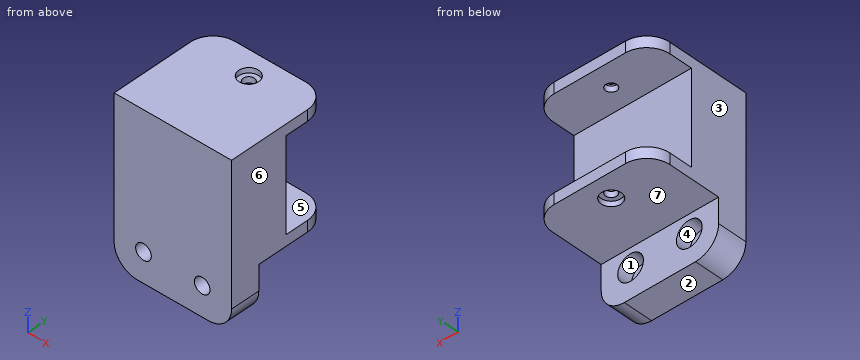
```python
from build123d import *

# Parameters (mm, degrees)
SKETCH1_W                                        = 50.8
SKETCH1_H                                        = 25.4
BOSS_EXTRUDE1_DEPTH                              = 25.4
CBORE_FOR_1_4_SOCKET_HEAD_CAP_SCREW1_D           = 6.7564
CBORE_FOR_1_4_SOCKET_HEAD_CAP_SCREW1_CBORE_D     = 11.1125
CBORE_FOR_1_4_SOCKET_HEAD_CAP_SCREW1_CBORE_DEPTH = 19.05
SKETCH6_W                                        = 50.8
SKETCH6_H                                        = 4.7
BOSS_EXTRUDE2_DEPTH                              = 20
CBORE_FOR_M4_SBHCS1_D                            = 4.8
CBORE_FOR_M4_SBHCS1_CBORE_D                      = 8.6
CBORE_FOR_M4_SBHCS1_CBORE_DEPTH                  = 2.2
FILLET1_R                                        = 10
SKETCH15_W                                       = 50.8
SKETCH15_H                                       = 25.4
BOSS_EXTRUDE3_DEPTH                              = 20
SKETCH16_W                                       = 51.113320751
SKETCH16_H                                       = 27.993322013
CUT_EXTRUDE2_DEPTH                               = 12.7
SKETCH17_W                                       = 50.8
SKETCH17_H                                       = 12.7
CUT_EXTRUDE3_DEPTH                               = 20.7


with BuildPart() as part:
    # Sketch1 → Boss-Extrude1 (new body)
    with BuildSketch(Plane(origin=(0, 0, 0), x_dir=(1, 0, 0), z_dir=(0, 1, 0))):
        with Locations((2.315568022, 7.890743338)):
            Rectangle(SKETCH1_W, SKETCH1_H)
    extrude(amount=BOSS_EXTRUDE1_DEPTH)

    # CBORE for 1/4 Socket Head Cap Screw1 (through all)
    with Locations(Plane(origin=(0, 25.4, 0), x_dir=(1, 0, 0), z_dir=(0, 1, 0))):
        with Locations((-10.384431978, 7.890743338), (15.015568022, 7.890743338)):
            CounterBoreHole(CBORE_FOR_1_4_SOCKET_HEAD_CAP_SCREW1_D / 2, CBORE_FOR_1_4_SOCKET_HEAD_CAP_SCREW1_CBORE_D / 2, CBORE_FOR_1_4_SOCKET_HEAD_CAP_SCREW1_CBORE_DEPTH)

    # Sketch6 → Boss-Extrude2 (add)
    with BuildSketch(Plane(origin=(0, 25.4, 0), x_dir=(1, 0, 0), z_dir=(0, 1, 0))):
        with Locations((2.315568022, 18.240743338)):
            Rectangle(SKETCH6_W, SKETCH6_H)
    extrude(amount=BOSS_EXTRUDE2_DEPTH)

    # CBORE for M4 SBHCS1 (through all)
    with Locations(Plane.XY.offset(-15.890743338)):
        with Locations((2.315568022, 35.4)):
            CounterBoreHole(CBORE_FOR_M4_SBHCS1_D / 2, CBORE_FOR_M4_SBHCS1_CBORE_D / 2, CBORE_FOR_M4_SBHCS1_CBORE_DEPTH)

    # Fillet1
    fillet1_edges = [part.edges().sort_by_distance(p)[0] for p in [
        (27.715568022, 45.4, -18.240743338),
        (-23.084431978, 45.4, -18.240743338),
        (27.715568022, 12.7, 4.809256662),
        (-23.084431978, 12.7, 4.809256662),
    ]]
    fillet(fillet1_edges, radius=FILLET1_R)

    # Sketch15 → Boss-Extrude3 (add)
    with BuildSketch(Plane(origin=(0, 0, -20.590743338), x_dir=(-1, 0, 0), z_dir=(0, 0, -1))):
        with Locations((-2.315568022, 12.7)):
            Rectangle(SKETCH15_W, SKETCH15_H)
    extrude(amount=BOSS_EXTRUDE3_DEPTH)

    # Sketch16 → Cut-Extrude2 (cut)
    with BuildSketch(Plane(origin=(0, 25.4, 0), x_dir=(1, 0, 0), z_dir=(0, 1, 0))):
        with Locations((2.472228398, 1.894082332)):
            Rectangle(SKETCH16_W, SKETCH16_H)
    extrude(amount=-CUT_EXTRUDE2_DEPTH, mode=Mode.SUBTRACT)

    # Mirror1: part across plane


with BuildPart() as part_1:
    add(part.part)
    add(part.part.mirror(Plane(origin=(0, 0, -40.590743338), x_dir=(1, 0, 0), z_dir=(0, 0, -1))))

    # Sketch17 → Cut-Extrude3 (cut)
    with BuildSketch(Plane.XY.offset(4.809256662)):
        with Locations((2.315568022, 6.35)):
            Rectangle(SKETCH17_W, SKETCH17_H)
    extrude(amount=-CUT_EXTRUDE3_DEPTH, mode=Mode.SUBTRACT)


solid = part_1.part
```
Source: CAD feature listing. Evaluate the final solid. Frame: model axes, mm. Face numbers are marked on the shaded views. A direction names the side the tool comes from. Round coordinates to 2 decimals unless told otherwise and drop trailing zeros. Loops run counter-clockwise (first coordinate to the right, second up) from the corner with the lowest first, then second, coordinate; pieces in that order, holes last.
(1) Contact query for flat-ended pins moving along their axis: pin 1 Ø10 at (x, y) = (4.5, 25) entering from -Z; pin 2 Ø4.5 at (x, y) = (2.32, 35.4) entering from +Z; pin 3 Ø16.5 at (x, z) = (4, -75) entering from +Y; pin 4 Ø7.5 at (x, y) = (2.32, 35.4) entering from -Z. Output: stop coordinate, or through.
From the geometry:
pin 1: stops at z = -65.29
pin 2: passes through
pin 3: stops at y = 12.7
pin 4: stops at z = -63.09
(2) Section query A-A (z = -64). Output: boundary loops of the cut face in (x, y), and give its area (3 significant figures).
From the geometry:
outline: (-23.08, 0) - (27.72, 0) - (27.72, 35.4) arc R10 ccw to (17.72, 45.4) - (-13.08, 45.4) arc R10 ccw to (-23.08, 35.4) - close; hole circle Ø8.6 at (2.32, 35.4)
area: 2,210 mm2
(3) Section query D-D (y = 14.5). Output: boundary loops of the cut face in (x, z).
From the geometry:
outline: (-23.08, -65.29) - (27.72, -65.29) - (27.72, -15.89) - (-23.08, -15.89) - close
(4) Section query B-B (x = -1). Output: boundary loops of the cut face in (y, z), and give its area (3 significant figures).
From the geometry:
outline: (0, -85.99) - (12.7, -85.99) - (12.7, -65.29) - (32.66, -65.29) - (32.66, -63.09) - (38.14, -63.09) - (38.14, -65.29) - (45.4, -65.29) - (45.4, -60.59) - (25.4, -60.59) - (25.4, -20.59) - (45.4, -20.59) - (45.4, -15.89) - (38.14, -15.89) - (38.14, -18.09) - (32.66, -18.09) - (32.66, -15.89) - (0, -15.89) - close
area: 1,680 mm2
(5) Material intervals for probe 1 along Z at (x, y) = (-16, 32); probe 2 along Z at (x, y) = (1, 33); probe 3 along Y at (x, z) = (10, -39), sorted ascending.
From the geometry:
probe 1: z = -65.29 to -60.59, -20.59 to -15.89
probe 2: z = -63.09 to -60.59, -20.59 to -18.09
probe 3: y = 0 to 25.4
(6) Pull-direction query (X, two-part tool) for the marked faces 1, 2, 3 and 4; classes: +X half, -X half, draft (parallel to the pull), parting line (faces both ways), or undercut.
From the geometry:
face 1: undercut
face 2: draft
face 3: -X half
face 4: undercut
(7) Section query C-C (z = -22.5). Output: boundary loops of the cut face in (x, y).
From the geometry:
outline: (-23.08, 0) - (27.72, 0) - (27.72, 25.4) - (-23.08, 25.4) - close
(8) Access query for the marked faces 5, 6 and 7. Directions: +Z, -Z, +X, -X, +Y, -Y. A direction counts if a zero-diameter tool reaches every point of the face in a straight line with its end or side. Return the directions, or none.
From the geometry:
face 5: +X, -X, +Y
face 6: +Z, -Z, +X, +Y, -Y
face 7: -Z, +X, -X, +Y
